```python
from build123d import *

# Parameters (mm, degrees)
SKETCH1_W           = 260
SKETCH1_H           = 120
BOSS_EXTRUDE1_DEPTH = 190
SHELL1_T            = 15
SKETCH2_R           = 15
CUT_EXTRUDE1_DEPTH  = 260.615099715
SKETCH3_R           = 23.5
CUT_EXTRUDE2_DEPTH  = 260.615099715
SKETCH4_R           = 2
CUT_EXTRUDE3_DEPTH  = 260.615099715


with BuildPart() as part:
    # Sketch1 → Boss-Extrude1 (new body)
    with BuildSketch(Plane(origin=(0, 0, 0), x_dir=(1, 0, 0), z_dir=(0, 1, 0))):
        Rectangle(SKETCH1_W, SKETCH1_H)
    extrude(amount=BOSS_EXTRUDE1_DEPTH)

    # Shell1 (no face opened: a closed hollow body)
    add(offset(amount=-SHELL1_T, mode=Mode.PRIVATE), mode=Mode.SUBTRACT)

    # Sketch2 → Cut-Extrude1 (cut, through all)
    with BuildSketch(Plane.XY.offset(60)):
        with Locations((-35, 95)):
            Circle(SKETCH2_R)
        with Locations((67, 95)):
            Circle(SKETCH2_R)
    extrude(amount=-CUT_EXTRUDE1_DEPTH, mode=Mode.SUBTRACT)

    # Sketch3 → Cut-Extrude2 (cut, through all)
    with BuildSketch(Plane.XY.offset(60)):
        with Locations((-35, 95)):
            Circle(SKETCH3_R)
        with Locations((67, 95)):
            Circle(SKETCH3_R)
    extrude(amount=-CUT_EXTRUDE2_DEPTH, mode=Mode.SUBTRACT)

    # Sketch4 → Cut-Extrude3 (cut, through all)
    with BuildSketch(Plane.XY.offset(60)):
        with Locations((36, 95)):
            Circle(SKETCH4_R)
        with Locations((67, 126)):
            Circle(SKETCH4_R)
        with Locations((98, 95)):
            Circle(SKETCH4_R)
        with Locations((67, 64)):
            Circle(SKETCH4_R)
        with Locations((-4, 95)):
            Circle(SKETCH4_R)
        with Locations((-35, 64)):
            Circle(SKETCH4_R)
        with Locations((-66, 95)):
            Circle(SKETCH4_R)
        with Locations((-35, 126)):
            Circle(SKETCH4_R)
    extrude(amount=-CUT_EXTRUDE3_DEPTH, mode=Mode.SUBTRACT)


solid = part.part
```
Geometry check sheet. Reference: the model listing, model coordinates, mm. A direction names the side the tool comes from. Coordinates: 2 decimals unless noted, no trailing zeros. Write each loop counter-clockwise with the first axis right and the second up, starting at its lowest first coordinate (ties: lowest second). Pieces come first, ordered by that corner, then holes. Notation, with made-up numbers: M 59.25,-8.75 L 83.25,-8.75 A12 ccw 83.25,3.25 Z; hole C 29,-17 d11. An arc over 180 degrees is marked long. Answer as a JSON object with one key per item and string values.
1. Go/stop test with a flat-tipped pin: pin 1 Ø5 at (x, y) = (98, 95) entering from -Z. Record where the tip stops, or that it passes through.
Answers below:
{"pin 1": "stops at z = -60"}
2. Section check A-A, the plane x = 14.5. Enter the section's corners in (y, z).
Answers below:
{"outline": "M 0,-60 L 190,-60 L 190,60 L 0,60 Z; hole M 15,-45 L 175,-45 L 175,45 L 15,45 Z"}
3. Tool access check on faces 1 (the cylindrical face through (-24.16, 74.15, -52.4)), 2 (the flat face through (-115, 94, 1)). Record the directions out of +Z, -Z, +X, -X, +Y, -Y that give a thin tool (end or side, any length) a straight path to the whole face; none if there is none.
Answers below:
{"face 1": "+Z, -Z", "face 2": "none"}
4. Section check C-C, the plane y = 109. Enter the section's corners in (x, z).
Answers below:
{"outline": "M -130,-60 L -53.87,-60 L -53.87,-45 L -115,-45 L -115,45 L -53.87,45 L -53.87,60 L -130,60 Z; M -16.13,-60 L 48.13,-60 L 48.13,-45 L -16.13,-45 Z; M -16.13,45 L 48.13,45 L 48.13,60 L -16.13,60 Z; M 85.87,-60 L 130,-60 L 130,60 L 85.87,60 L 85.87,45 L 115,45 L 115,-45 L 85.87,-45 Z"}
5. Section check D-D, the plane x = -27. Enter the section's corners in (y, z).
Answers below:
{"outline": "M 0,-60 L 72.9,-60 L 72.9,-45 L 15,-45 L 15,45 L 72.9,45 L 72.9,60 L 0,60 Z; M 117.1,-60 L 190,-60 L 190,60 L 117.1,60 L 117.1,45 L 175,45 L 175,-45 L 117.1,-45 Z"}
6. Draft check along Z on faces 3 (the flat face through (-2, 94, 60)), 4 (the flat face through (-2, 94, 45)), 5 (the cylindrical face through (-24.16, 74.15, 52.6)). Enter one of: released by +Z, released by -Z, zero draft, split by the parting line, or undercut.
Answers below:
{"face 3": "released by +Z", "face 4": "undercut", "face 5": "zero draft"}
7. Section check B-B, the plane z = 11. Enter the section's corners in (x, y).
Answers below:
{"outline": "M -130,0 L 130,0 L 130,190 L -130,190 Z; hole M -115,15 L 115,15 L 115,175 L -115,175 Z"}
8. Scan lines: L1, parallel to Y at x = -35, z = 51; L2, parallel to X at y = 125.5, z = -46.5; L3, parallel to Z at x = -11, y = 58. Record each from-to range of solid material in increasing order.
Answers below:
{"L1": "y = 0 to 62, 66 to 71.5, 118.5 to 124, 128 to 190", "L2": "x = -130 to -36.94, -33.06 to 65.06, 68.94 to 130", "L3": "z = -60 to -45, 45 to 60"}
